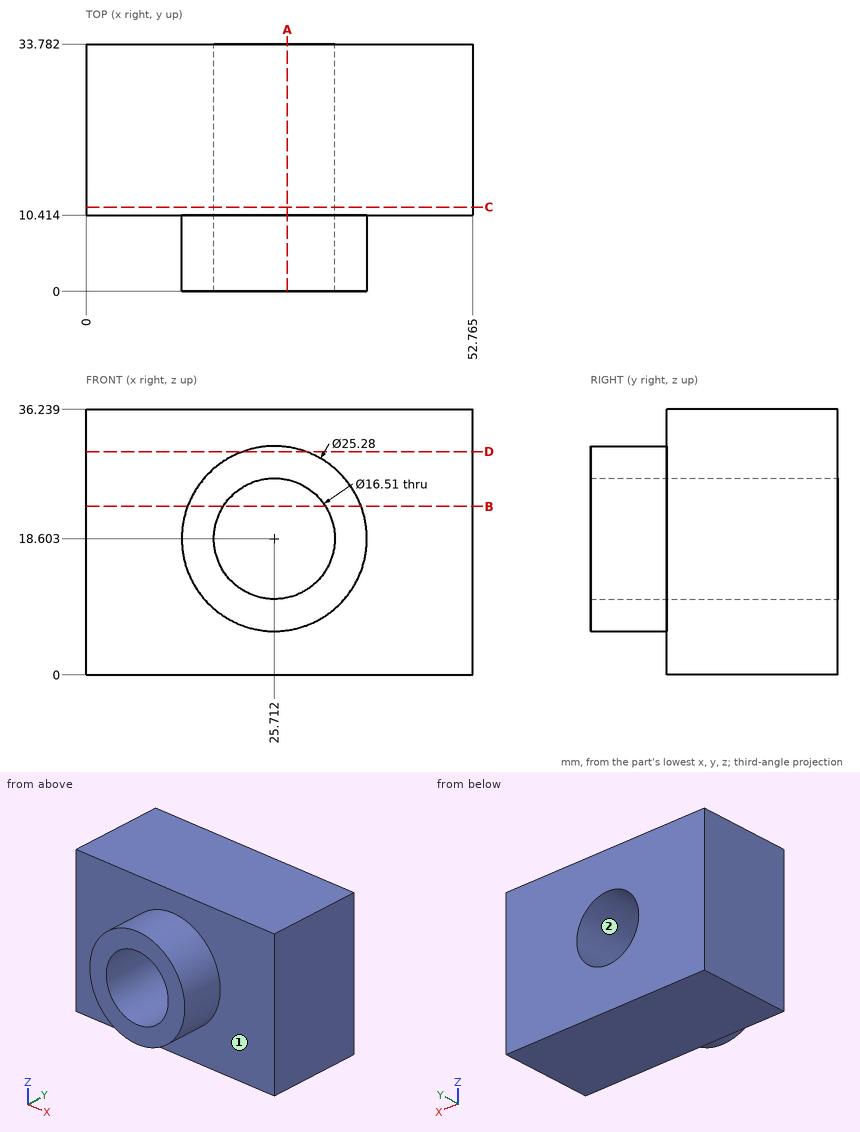
The drawing under review shows one solid part. Ordinate dimensions are in mm from its lowest x, y, z. A direction names the side the tool comes from. Round coordinates to 2 decimals unless told otherwise and drop trailing zeros. Write each loop counter-clockwise with the first axis right and the second up, starting at its lowest first coordinate (ties: lowest second). Pieces come first, ordered by that corner, then holes. Notation, with made-up numbers: (34, -30.5) - (63, -30.5) arc R27 ccw to (63, -9.5) - close; hole circle Ø4 at (73, 56.25). An arc over 180 degrees is marked (long way). Put each result on its own line as item: value.
Q1. Wall thickness on probe 1 along X at (y, z) = (18, 19) (1 decimal); probe 2 along Y at (x, z) = (5, 5); probe 3 along X at (y, z) = (7, 12) (1 decimal): over which ranges is each line inside the solid? List them lowest first.
Solved:
probe 1: x = 0 to 17.5, 34 to 52.8
probe 2: y = 10.41 to 33.78
probe 3: x = 14.9 to 20.8, 30.7 to 36.5
Q2. We need section A-A (x = 27.5). Give the boundary of the cut face in (y, z) (1 decimal).
Solved:
outline: (0, 6.1) - (10.4, 6.1) - (10.4, 0) - (33.8, 0) - (33.8, 10.5) - (0, 10.5) - close; (0, 26.7) - (33.8, 26.7) - (33.8, 36.2) - (10.4, 36.2) - (10.4, 31.1) - (0, 31.1) - close
Q3. Machinability: for the marked faces 1 and 2, which of the approach directions +Z, -Z, +X, -X, +Y, -Y give a long, thin tool a straight path to every point of the face, cutting with its end or side? Answer none if there is none.
Solved:
face 1: -Y
face 2: +Y, -Y
Q4. We need section B-B (z = 23). Give the boundary of the cut face in (x, y) (1 decimal).
Solved:
outline: (0, 10.4) - (13.9, 10.4) - (13.9, 0) - (18.7, 0) - (18.7, 33.8) - (0, 33.8) - close; (32.7, 0) - (37.6, 0) - (37.6, 10.4) - (52.8, 10.4) - (52.8, 33.8) - (32.7, 33.8) - close
Q5. We need section C-C (y = 11.5). Give the boundary of the cut face in (x, z) (1 decimal), and give its area (3 significant figures).
Solved:
outline: (0, 0) - (52.8, 0) - (52.8, 36.2) - (0, 36.2) - close; hole circle Ø16.5 at (25.7, 18.6)
area: 1,700 mm2
Q6. Insertion check: pin 1 Ø10 at (x, y) = (14.5, 5) entering from +Z; pin 2 Ø4 at (x, y) = (21, 6.5) entering from +Z. Each pin has a flat end and moves straight along its axis. Give the tip position at first contact, or say it passes through.
Solved:
pin 1: stops at z = 29.61
pin 2: stops at z = 30.95
Q7. We need section D-D (z = 30.5). Give the boundary of the cut face in (x, y) (1 decimal).
Solved:
outline: (0, 10.4) - (21.4, 10.4) - (21.4, 0) - (30, 0) - (30, 10.4) - (52.8, 10.4) - (52.8, 33.8) - (0, 33.8) - close
